Source: CAD feature listing. Evaluate the final solid. Frame: model axes, mm. A direction names the side the tool comes from. Give positions to 0.01 mm unless a question says otherwise; leave off trailing zeros. Order: outer loops, then holes, each group sorted by start corner. A loop starts at its lowest first (then second) coordinate and runs counter-clockwise, first axis right, second up. Notation, with made-up numbers: (8.25, -24) -> (26.25, -24) arc R11 cw to (26.25, -6) -> close; hole circle Ø11 at (77.25, -26). An arc over 180 degrees is marked (long way). Answer in a Markdown table with one row per item.
```python
from build123d import *

# Parameters (mm, degrees)
EXTRUDE_1_DEPTH      = 7.75
EXTRUDE_1_DEPTH_BACK = 7.75
SKETCH_3_R           = 2
CUT_EXTRUDE_2_DEPTH  = 15.5
SKETCH_4_R           = 2
CUT_EXTRUDE_3_DEPTH  = 15.5
FILLET_1_R           = 7.75
CHAMFER_1_SIZE       = 1.5


with BuildPart() as part:
    # 草图1 → 凸台-拉伸1 (new, two sides: drawn at the far end of the back side and taken through both)
    with BuildSketch(Plane(origin=(0, 0, 0), x_dir=(0, 0, -1), z_dir=(1, 0, 0)).offset(-EXTRUDE_1_DEPTH_BACK)):
        with BuildLine():
            Line((-30, 0), (-3, 0))
            ThreePointArc((-3, 0), (-0.878679656, 0.878679656), (0, 3))
            Line((0, 3), (0, 30))
            Line((0, 30), (-2, 30))
            Line((-2, 30), (-2, 3))
            ThreePointArc((-2, 3), (-2.292893219, 2.292893219), (-3, 2))
            Line((-3, 2), (-30, 2))
            Line((-30, 2), (-30, 0))
        make_face()
    extrude(amount=EXTRUDE_1_DEPTH + EXTRUDE_1_DEPTH_BACK)

    # 草图3 → 切除-拉伸2 (cut)
    with BuildSketch(Plane(origin=(0, 2, 0), x_dir=(1, 0, 0), z_dir=(0, 1, 0))):
        with Locations(Location((0, -23, 0), (0, 0, 270))):
            Circle(SKETCH_3_R)
    extrude(amount=-CUT_EXTRUDE_2_DEPTH, mode=Mode.SUBTRACT)

    # 草图4 → 切除-拉伸3 (cut)
    with BuildSketch(Plane.XY.offset(2)):
        with Locations((0, 23)):
            Circle(SKETCH_4_R)
    extrude(amount=-CUT_EXTRUDE_3_DEPTH, mode=Mode.SUBTRACT)

    # 圆角1
    fillet_1_edges = [part.edges().sort_by_distance(p)[0] for p in [
        (7.75, 30, 1),
        (-7.75, 30, 1),
        (7.75, 1, 30),
        (-7.75, 1, 30),
    ]]
    fillet(fillet_1_edges, radius=FILLET_1_R - 0.0001)  # a hair under: the kernel refuses the full size

    # 倒角1
    chamfer_1_edges = [part.edges().sort_by_distance(p)[0] for p in [
        (0, 2, 21),
        (-2, 23, 2),
    ]]
    chamfer(chamfer_1_edges, length=CHAMFER_1_SIZE)


solid = part.part
```
(1) Ray query, probe 1 along Z at (x, y) = (6.25, 13); probe 2 along Y at (x, z) = (0, 0.25). Return the intervals inside material, ascending.
A:
| item | result |
|---|---|
| probe 1 | z = 0 to 2 |
| probe 2 | y = 1.8 to 21, 25 to 30 |
(2) First-contact query: pin 1 Ø4.5 at (x, z) = (0.5, 12) entering from +Y; pin 2 Ø1.5 at (x, y) = (1, 9) entering from +Z. Flat tips, straight axial feed; report the tip coordinate or a pass-through.
A:
| item | result |
|---|---|
| pin 1 | stops at y = 2 |
| pin 2 | stops at z = 2 |
(3) Section query A-A (z = 23). Return the cut outline in (x, y), plus the area to 3 significant figures.
A:
| item | result |
|---|---|
| outline | (-7.71, 0) -> (-2, 0) -> (-2, 0.5) -> (-3.5, 2) -> (-7.71, 2) -> close; (2, 0) -> (7.71, 0) -> (7.71, 2) -> (3.5, 2) -> (2, 0.5) -> close |
| area | 20.6 mm^2 |
(4) Section query D-D (y = 7). Return the cut outline in (x, z), plus the area to 3 significant figures.
A:
| item | result |
|---|---|
| outline | (-7.75, 0) -> (7.75, 0) -> (7.75, 2) -> (-7.75, 2) -> close |
| area | 31.0 mm^2 |
(5) Section query C-C (x = 5.5). Return the cut outline in (y, z), plus the area to 3 significant figures.
A:
| item | result |
|---|---|
| outline | (0, 3) arc R3 ccw to (3, 0) -> (27.71, 0) -> (27.71, 2) -> (3, 2) arc R1 cw to (2, 3) -> (2, 27.71) -> (0, 27.71) -> close |
| area | 105 mm^2 |
(6) Pull-direction query (X, two-part tool) for faces 3 (the flat face through (0, 2, 16)), 4 (the cylindrical face through (-5.54, 27.67, 1.01)), 5 (the cylindrical face through (-1.2, 0.3, 21.4)); classes: +X half, -X half, draft (parallel to the pull), parting line (faces both ways), or undercut.
A:
| item | result |
|---|---|
| face 3 | draft |
| face 4 | -X half |
| face 5 | undercut |
(7) Access query for faces 1 (the cylindrical face through (5.42, 0.99, 27.79)), 2 (the flat face through (0, 14, 2)). Directions: +Z, -Z, +X, -X, +Y, -Y. A direction counts if a zero-diameter tool reaches every point of the face in a straight line with its end or side. Return the directions, or none.
A:
| item | result |
|---|---|
| face 1 | +Z, +X, +Y, -Y |
| face 2 | +Z, +X, -X, +Y |
